Autodesk Inventor part; units mm, degrees
ref_plane "YZ Plane" through (0, 0, 0) normal (1, 0, 0) x (0, 1, 0)
ref_plane "XZ Plane" through (0, 0, 0) normal (0, 1, 0) x (-1, 0, 0)
ref_plane "XY Plane" through (0, 0, 0) normal (0, 0, 1) x (1, 0, 0)
sketch "Sketch1" plane through (0, 0, 0) normal (0, 0, 1) x (1, 0, 0)
  line L0 (0, 0) -> (0, -12.7)
  line L1 (0, -12.7) -> (12.7, -12.7)
  line L2 (12.7, -12.7) -> (12.7, 0)
  line L3 (12.7, 0) -> (14.2875, 0)
  line L4 (12.7, -14.2875) -> (14.2875, -14.2875)
  line L5 (14.2875, -14.2875) -> (14.2875, 0)
  line L6 (0, 0) -> (-1.5875, 0)
  line L7 (-1.5875, 0) -> (-1.5875, -14.2875)
  line L8 (-1.5875, -14.2875) -> (12.7, -14.2875)
  dimension "d0" = 12.7
  dimension "d2" = 1.5875
  dimension "d3" = 1.5875
  dimension "d4" = 1.5875
extrude "Extrusion1" add sketch "Sketch1" along normal blind 381
properties part number "BackLiftProtoPart7"
Geometry: final body of the model. Coordinates: model frame, mm. A direction names the side the tool comes from. Round coordinates to 2 decimals unless told otherwise and drop trailing zeros. Loops run counter-clockwise (first coordinate to the right, second up) from the corner with the lowest first, then second, coordinate; pieces in that order, holes last. Notation, with made-up numbers: (-38, 75.25) -> (5, 75.25) arc R21 cw to (5, 104.25) -> close; hole circle Ø3 at (59.5, 34). An arc over 180 degrees is marked (long way). Write each question's results on one line, items separated by ' | '.
Item 1: Cut plane C-C on x = 6.25. Return the cut outline in (y, z).
Answers below:
outline: (-14.29, 0) -> (-12.7, 0) -> (-12.7, 381) -> (-14.29, 381) -> close
Item 2: Pull-direction query (X, two-part tool) for faces 3 (the face through (0, -6, 188)), 4 (the face through (6, -13, 381)), 5 (the face through (-1.588, -7, 188)), 6 (the face through (12.7, -6, 188)); classes: pulls with the +X half, pulls with the -X half, needs draft (parallel to the pull), parting line crosses it, or undercut.
Answers below:
face 3: undercut | face 4: needs draft | face 5: pulls with the -X half | face 6: undercut
Item 3: Cut plane B-B on z = 111. Return the cut outline in (x, y).
Answers below:
outline: (-1.59, -14.29) -> (14.29, -14.29) -> (14.29, 0) -> (12.7, 0) -> (12.7, -12.7) -> (0, -12.7) -> (0, 0) -> (-1.59, 0) -> close
Item 4: Line query: probe 1 along X at (y, z) = (-1.75, 174); probe 2 along Y at (x, z) = (1.25, 270.5). Output: solid intervals per line, ascending. Write a range as [from, to].
Answers below:
probe 1: x = [-1.59, 0], [12.7, 14.29] | probe 2: y = [-14.29, -12.7]
Item 5: Pin query (flat end, axial travel): pin 1 Ø4 at (x, z) = (10, 164) entering from +Y. Return the tip coordinate at first contact, or that it passes through.
Answers below:
pin 1: stops at y = -12.7
Item 6: Cut plane A-A on y = -6. Return the cut outline in (x, z).
Answers below:
outline: (-1.59, 0) -> (0, 0) -> (0, 381) -> (-1.59, 381) -> close; (12.7, 0) -> (14.29, 0) -> (14.29, 381) -> (12.7, 381) -> close
Item 7: Set-up query: faces 1 (the face through (6, -13, 0)), 2 (the face through (6, -12.7, 188)). Return all of +Z, -Z, +X, -X, +Y, -Y with unobstructed straight access to the full face (end or side cutting, diameter ignored); none if empty.
Answers below:
face 1: -Z, +X, -X, +Y, -Y | face 2: +Z, -Z, +Y
